Could you check a few things on this model? Use its own coordinates, in mm. Face numbers are marked on the shaded views. A direction names the side the tool comes from. Round coordinates to 2 decimals unless told otherwise and drop trailing zeros. Write each loop counter-clockwise with the first axis right and the second up, starting at its lowest first coordinate (ties: lowest second). Pieces come first, ordered by that corner, then holes. Notation, with made-up numbers: (39, 43) -> (68, 43) arc R14 ccw to (68, 58) -> close; hole circle Ø8 at (50.5, 47.25). An arc over 180 degrees is marked (long way). Return JSON: item names as keys, results as strings.
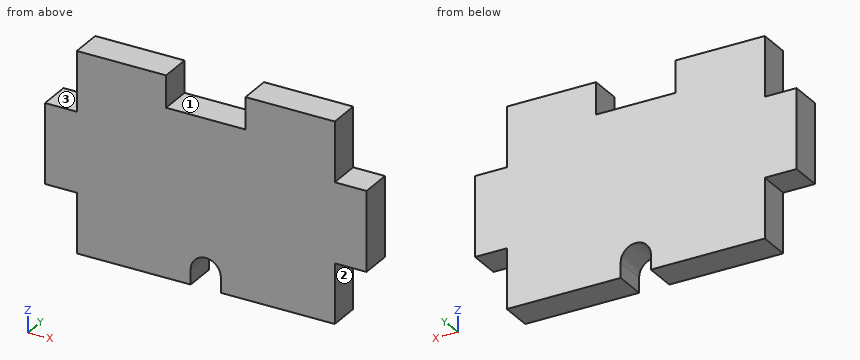
from build123d import *

# Parameters (mm, degrees)
SKETCH1_W           = 32.5
SKETCH1_H           = 25
BOSS_EXTRUDE1_DEPTH = 4
SKETCH2_R           = 1.9
SKETCH2_W           = 3.8
SKETCH2_H           = 1.9
CUT_EXTRUDE5_DEPTH  = 5
SKETCH3_W           = 4
SKETCH3_H           = 10
BOSS_EXTRUDE2_DEPTH = 4
SKETCH4_W           = 10
SKETCH4_H           = 4
CUT_EXTRUDE6_DEPTH  = 5


with BuildPart() as part:
    # Sketch1 → Boss-Extrude1 (new body)
    with BuildSketch(Plane(origin=(0, 0, 0), x_dir=(1, 0, 0), z_dir=(0, 1, 0))):
        with Locations((16.25, -12.5)):
            Rectangle(SKETCH1_W, SKETCH1_H)
    extrude(amount=BOSS_EXTRUDE1_DEPTH)

    # Sketch2 → Cut-Extrude5 (cut, through all)
    with BuildSketch(Plane(origin=(0, 4, 0), x_dir=(1, 0, 0), z_dir=(0, 1, 0))):
        with Locations((16.25, -1.9)):
            Circle(SKETCH2_R)
        with Locations((16.25, -0.95)):
            Rectangle(SKETCH2_W, SKETCH2_H)
    extrude(amount=-CUT_EXTRUDE5_DEPTH, mode=Mode.SUBTRACT)

    # Sketch3 → Boss-Extrude2 (add, through all)
    with BuildSketch(Plane(origin=(0, 4, 0), x_dir=(1, 0, 0), z_dir=(0, 1, 0))):
        with Locations((-2, -12.5)):
            Rectangle(SKETCH3_W, SKETCH3_H)
        with Locations((34.5, -12.5)):
            Rectangle(SKETCH3_W, SKETCH3_H)
    extrude(amount=-BOSS_EXTRUDE2_DEPTH)

    # Sketch4 → Cut-Extrude6 (cut, through all)
    with BuildSketch(Plane(origin=(0, 4, 0), x_dir=(1, 0, 0), z_dir=(0, 1, 0))):
        with Locations((16.25, -23)):
            Rectangle(SKETCH4_W, SKETCH4_H)
    extrude(amount=-CUT_EXTRUDE6_DEPTH, mode=Mode.SUBTRACT)


solid = part.part
1) I want a section at C-C, the plane x = 34. Please give me the cut outline in (y, z), and give its area (3 significant figures).
Return value:
{"outline": "(0, 7.5) -> (4, 7.5) -> (4, 17.5) -> (0, 17.5) -> close", "area": "40.0 mm²"}
2) Will these pins go through, and if not, where does the flat tip stop? pin 1 Ø1.2 at (y, z) = (2.5, 23) entering from +X; pin 2 Ø2 at (x, y) = (18.5, 2.5) entering from +Z; pin 3 Ø1.2 at (x, y) = (35, 2.5) entering from +Z; pin 4 Ø1 at (x, z) = (2.5, 6) entering from -Y.
Return value:
{"pin 1": "x = 32.5", "pin 2": "z = 21", "pin 3": "z = 17.5", "pin 4": "y = 0"}
3) I want a section at B-B, the plane z = 6.25. Please give me the cut outline in (x, y).
Return value:
{"outline": "(0, 0) -> (32.5, 0) -> (32.5, 4) -> (0, 4) -> close"}
4) I want a section at A-A, the plane y = 2.5. Please give me the cut outline in (x, z).
Return value:
{"outline": "(-4, 7.5) -> (0, 7.5) -> (0, 0) -> (14.35, 0) -> (14.35, 1.9) arc R1.9 cw to (18.15, 1.9) -> (18.15, 0) -> (32.5, 0) -> (32.5, 7.5) -> (36.5, 7.5) -> (36.5, 17.5) -> (32.5, 17.5) -> (32.5, 25) -> (21.25, 25) -> (21.25, 21) -> (11.25, 21) -> (11.25, 25) -> (0, 25) -> (0, 17.5) -> (-4, 17.5) -> close"}
5) If I drill on probe 1 along X at (y, z) = (1.3, 22); probe 2 along Z at (x, y) = (-1, 1.4); probe 3 along Z at (x, y) = (12, 0.3), over which ranges is the centre line in solid material (lowest first)? Write a range as [from, to].
Return value:
{"probe 1": "[0, 11.25], [21.25, 32.5]", "probe 2": "[7.5, 17.5]", "probe 3": "[0, 21]"}
6) For the marked faces 1, 2 and 3, which set-ups out of +Z, -Z, +X, -X, +Y, -Y let a thin tool reach every point of the face, with its end or its side?
Return value:
{"face 1": "+Z, +Y, -Y", "face 2": "-Z, +X, +Y, -Y", "face 3": "+Z, -X, +Y, -Y"}
